Answer from the drawing. Dimensions are ordinates in mm from the lowest x, y and z of the part. Give positions to 0.01 mm unless a question says otherwise; leave off trailing zeros. Loops run counter-clockwise (first coordinate to the right, second up) from the corner with the lowest first, then second, coordinate; pieces in that order, holes last.
(1) Find section A-A, the plane x = 21. Write down the section's boundary in (y, z).
(2) Find section B-B, the plane z = 44. Write down the section's boundary in (x, y), then the cut area to 3 significant figures.
(3) Find section C-C, the plane y = 0.7. Write down the section's boundary in (x, z), then the cut area to 3 significant figures.
(4) Find section D-D, the plane z = 77.5. Write down the section's boundary in (x, y).
(5) This flat-tipped pin is pushed along its axis until it touches: P1, Ø1.7, axis at x = 6, z = 77.5, coming from the +Y side. Where does it stop, or does it pass through?
(6) Straight lines are drawn through the part: probe 1 along X at (y, z) = (0.8, 55); probe 2 along Z at (x, y) = (5.25, 0.6); probe 3 along X at (y, z) = (2.8, 13). For each, find the intervals that lie inside material, in ascending order.
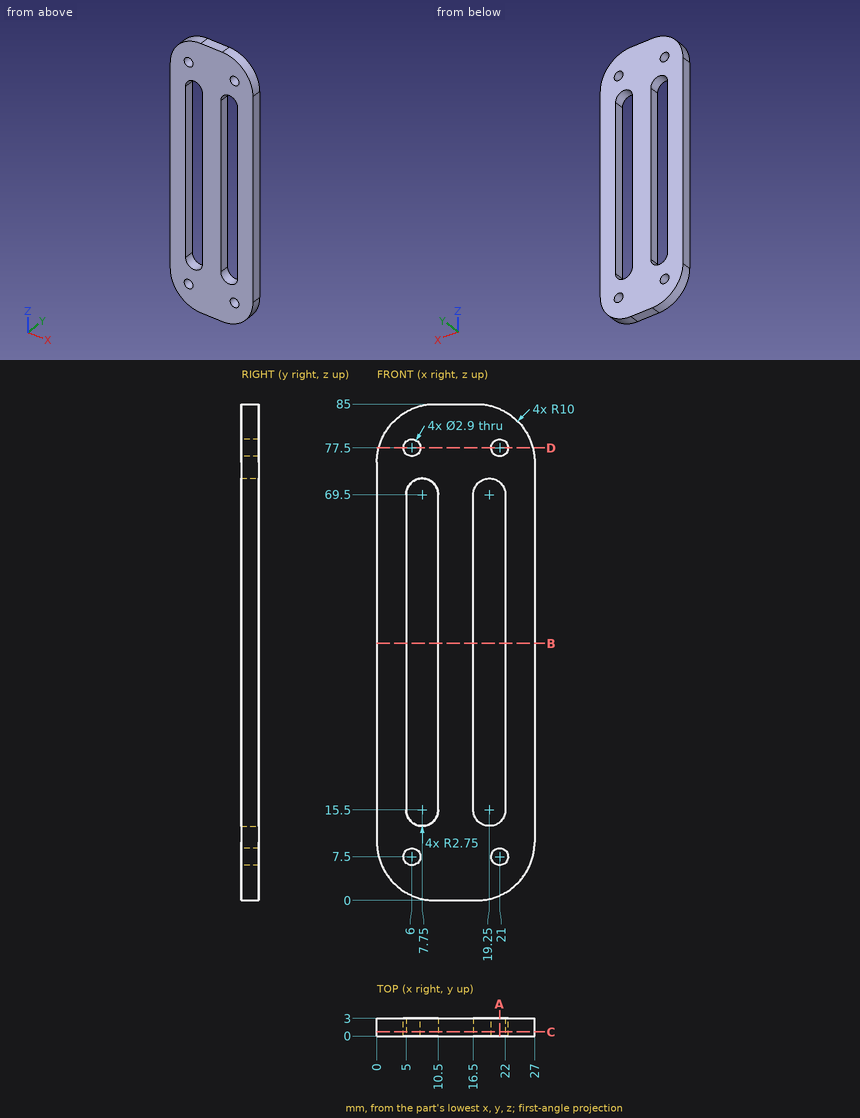
Entries:
1. outline: (0, 0.83) - (3, 0.83) - (3, 6.05) - (0, 6.05) - close; (0, 8.95) - (3, 8.95) - (3, 13.38) - (0, 13.38) - close; (0, 71.62) - (3, 71.62) - (3, 76.05) - (0, 76.05) - close; (0, 78.95) - (3, 78.95) - (3, 84.17) - (0, 84.17) - close
2. outline: (0, 0) - (5, 0) - (5, 3) - (0, 3) - close; (10.5, 0) - (16.5, 0) - (16.5, 3) - (10.5, 3) - close; (22, 0) - (27, 0) - (27, 3) - (22, 3) - close
2. area: 48.0 mm2
3. outline: (0, 10) arc R10 ccw to (10, 0) - (17, 0) arc R10 ccw to (27, 10) - (27, 75) arc R10 ccw to (17, 85) - (10, 85) arc R10 ccw to (0, 75) - close; hole circle Ø2.9 at (6, 7.5); hole circle Ø2.9 at (6, 77.5); hole (5, 15.5) arc R2.75 ccw to (10.5, 15.5) - (10.5, 69.5) arc R2.75 ccw to (5, 69.5) - close; hole (16.5, 15.5) arc R2.75 ccw to (22, 15.5) - (22, 69.5) arc R2.75 ccw to (16.5, 69.5) - close; hole circle Ø2.9 at (21, 7.5); hole circle Ø2.9 at (21, 77.5)
3. area: 1,540 mm2
4. outline: (0.32, 0) - (4.55, 0) - (4.55, 3) - (0.32, 3) - close; (7.45, 0) - (19.55, 0) - (19.55, 3) - (7.45, 3) - close; (22.45, 0) - (26.68, 0) - (26.68, 3) - (22.45, 3) - close
5. P1: passes through
6. probe 1: x = 0 to 5, 10.5 to 16.5, 22 to 27
6. probe 2: z = 1.2 to 6.26, 8.74 to 14.35, 70.65 to 76.26, 78.74 to 83.8
6. probe 3: x = 0 to 6.6, 8.9 to 18.1, 20.4 to 27
